```python
from build123d import *

# Parameters (mm, degrees)
BOSS_EXTRUDE1_DEPTH         = 3.302
F_1_4_0_13_DIAMETER_HOLE1_D = 3.302


with BuildPart() as part:
    # Sketch1 → Boss-Extrude1 (new body)
    with BuildSketch(Plane.XY):
        with BuildLine():
            Line((35.687, -3.175), (-35.687, -3.175))
            ThreePointArc((-35.687, -3.175), (-38.862, 0), (-35.687, 3.175))
            Line((-35.687, 3.175), (35.687, 3.175))
            ThreePointArc((35.687, 3.175), (38.862, 0), (35.687, -3.175))
        make_face()
    extrude(amount=-BOSS_EXTRUDE1_DEPTH)

    # 1/4 (0.13) Diameter Hole1 (through all)
    with Locations(Plane.XY):
        with Locations((-32.512, 0), (32.512, 0)):
            Hole(F_1_4_0_13_DIAMETER_HOLE1_D / 2)


solid = part.part
```
Could you check a few things on this model? Use its own coordinates, in mm. Round coordinates to 2 decimals unless told otherwise and drop trailing zeros. Loops run counter-clockwise (first coordinate to the right, second up) from the corner with the lowest first, then second, coordinate; pieces in that order, holes last. Notation, with made-up numbers: (40.25, -37.75) - (86.25, -37.75) arc R20 ccw to (86.25, -17.75) - close; hole circle Ø3 at (3, 64.5). An arc over 180 degrees is marked (long way). Answer in a Markdown table with one row per item. Add a question column.
(1) If we section it at C-C (z = -0.55): Please give me the cut outline in (x, y) (3 decimals), plus the area to 3 significant figures.
(2) If we mould it in two halves opening along X, with no side actions, what happens to faces 1 (the face through (0, -3.175, -2)), 2 (the face through (-34.087, 0.496, -1.674)), 3 (the face through (-38.86, -0.07, -1.63))? For each: pulls with the +X half, pulls with the -X half, needs draft (parallel to the pull), parting line crosses it, or undercut.
(3) If we section it at A-A (y = 0): Please give me the cut outline in (x, z), plus the area to 3 significant figures.
(4) If we section it at B-B (x = 32): Please give me the cut outline in (y, z) (3 decimals), plus the area to 3 significant figures.
(5) I'm going to push a flat-ended pin straight in: pin 1 (2 mm diameter, centred on x = 32.512, y = 0, fed in from +Z). Where does the tip first touch, or does it pass through?
(6) I need wall thicknesses on line 1 along X through (y, z) = (0.25, -2.8); line 2 along X through (y, z) = (-1.25, -2.6); line 3 along X through (y, z) = (2.75, -2.65). Which ranges of each line are inside material? Lowest first, please.
Model answer:
| question | item | result |
|---|---|---|
| 1 | outline | (-35.687, -3.175) - (35.687, -3.175) arc R3.175 ccw to (35.687, 3.175) - (-35.687, 3.175) arc R3.175 ccw to start; hole circle Ø3.302 at (-32.512, 0); hole circle Ø3.302 at (32.512, 0) |
| 1 | area | 468 mm² |
| 2 | face 1 | needs draft |
| 2 | face 2 | undercut |
| 2 | face 3 | pulls with the -X half |
| 3 | outline | (-38.86, -3.3) - (-34.16, -3.3) - (-34.16, 0) - (-38.86, 0) - close; (-30.86, -3.3) - (30.86, -3.3) - (30.86, 0) - (-30.86, 0) - close; (34.16, -3.3) - (38.86, -3.3) - (38.86, 0) - (34.16, 0) - close |
| 3 | area | 235 mm² |
| 4 | outline | (-3.175, -3.302) - (-1.57, -3.302) - (-1.57, 0) - (-3.175, 0) - close; (1.57, -3.302) - (3.175, -3.302) - (3.175, 0) - (1.57, 0) - close |
| 4 | area | 10.6 mm² |
| 5 | pin 1 | passes through |
| 6 | line 1 | x = -38.85 to -34.14, -30.88 to 30.88, 34.14 to 38.85 |
| 6 | line 2 | x = -38.61 to -33.59, -31.43 to 31.43, 33.59 to 38.61 |
| 6 | line 3 | x = -37.27 to 37.27 |
